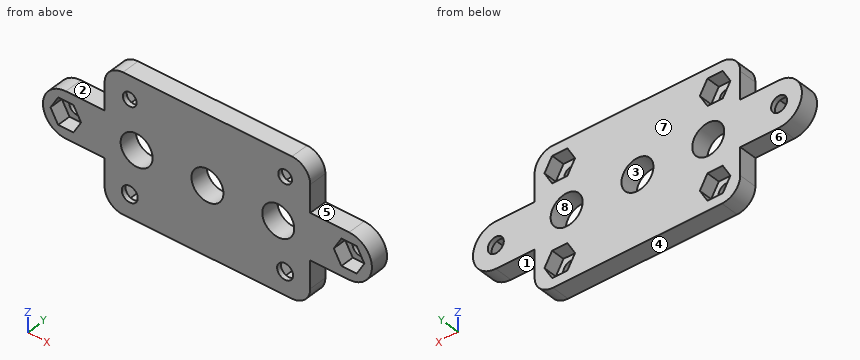
from build123d import *

# Parameters (mm, degrees)
ESBO_O2_R                = 1.75
ESBO_O2_R_2              = 1.5
ESBO_O2_R_3              = 3.5
RESSALTO_EXTRUS_O1_DEPTH = 4
CORTE_EXTRUS_O1_DEPTH    = 3
FILETE1_R                = 4
CORTE_EXTRUS_O2_DEPTH    = 3


with BuildPart() as part:
    # Esboço2 → Ressalto-extrusão1 (new body)
    with BuildSketch(Plane(origin=(0, 0, 0), x_dir=(1, 0, 0), z_dir=(0, 1, 0))):
        with BuildLine():
            Line((-22.5, -15), (22.5, -15))
            Line((22.5, -15), (22.5, -5))
            Line((22.5, -5), (31, -5))
            ThreePointArc((31, -5), (36, 0), (31, 5))
            Line((31, 5), (22.5, 5))
            Line((22.5, 5), (22.5, 15))
            Line((22.5, 15), (-22.5, 15))
            Line((-22.5, 15), (-22.5, 5))
            Line((-22.5, 5), (-31, 5))
            ThreePointArc((-31, 5), (-36, 0), (-31, -5))
            Line((-31, -5), (-22.5, -5))
            Line((-22.5, -5), (-22.5, -15))
        make_face()
        with Locations(Location((17, 10, 0), (0, 0, 270))):
            Circle(ESBO_O2_R, mode=Mode.SUBTRACT)
        with Locations(Location((17, -10, 0), (0, 0, 270))):
            Circle(ESBO_O2_R_2, mode=Mode.SUBTRACT)
        with Locations(Location((-17, -10, 0), (0, 0, 90))):
            Circle(ESBO_O2_R_2, mode=Mode.SUBTRACT)
        with Locations(Location((-17, 10, 0), (0, 0, 90))):
            Circle(ESBO_O2_R, mode=Mode.SUBTRACT)
        with Locations(Location((31, 0, 0), (0, 0, 270))):
            Circle(ESBO_O2_R, mode=Mode.SUBTRACT)
        with Locations(Location((-31, 0, 0), (0, 0, 90))):
            Circle(ESBO_O2_R, mode=Mode.SUBTRACT)
        with Locations(Location((0, 0, 0), (0, 0, 270))):
            Circle(ESBO_O2_R_3, mode=Mode.SUBTRACT)
        with Locations(Location((15.5, 0, 0), (0, 0, 270))):
            Circle(ESBO_O2_R_3, mode=Mode.SUBTRACT)
        with Locations(Location((-15.5, 0, 0), (0, 0, 90))):
            Circle(ESBO_O2_R_3, mode=Mode.SUBTRACT)
    extrude(amount=RESSALTO_EXTRUS_O1_DEPTH)

    # Esboço3 → Corte-extrusão1 (cut)
    with BuildSketch(Plane(origin=(0, 4, 0), x_dir=(1, 0, 0), z_dir=(0, 1, 0))):
        Polygon((-13.651368439, 10), (-15.325684219, 12.9), (-18.674315781, 12.9), (-20.348631561, 10), (-18.674315781, 7.1), (-15.325684219, 7.1), align=None)
        Polygon((-20.348631561, -10), (-18.674315781, -7.1), (-15.325684219, -7.1), (-13.651368439, -10), (-15.325684219, -12.9), (-18.674315781, -12.9), align=None)
        Polygon((18.674315781, -7.1), (15.325684219, -7.1), (13.651368439, -10), (15.325684219, -12.9), (18.674315781, -12.9), (20.348631561, -10), align=None)
        Polygon((15.325684219, 7.1), (13.651368439, 10), (15.325684219, 12.9), (18.674315781, 12.9), (20.348631561, 10), (18.674315781, 7.1), align=None)
    extrude(amount=-CORTE_EXTRUS_O1_DEPTH, mode=Mode.SUBTRACT)

    # Filete1
    filete1_edges = [part.edges().sort_by_distance(p)[0] for p in [
        (22.5, 2, 15),
        (-22.5, 2, 15),
        (-22.5, 2, -15),
        (22.5, 2, -15),
    ]]
    fillet(filete1_edges, radius=FILETE1_R)

    # Esboço6 → Corte-extrusão2 (cut)
    with BuildSketch(Plane.XZ):
        Polygon((-27.651368439, 0), (-29.325684219, 2.9), (-32.674315781, 2.9), (-34.348631561, 0), (-32.674315781, -2.9), (-29.325684219, -2.9), align=None)
        Polygon((29.325684219, -2.9), (27.651368439, 0), (29.325684219, 2.9), (32.674315781, 2.9), (34.348631561, 0), (32.674315781, -2.9), align=None)
    extrude(amount=-CORTE_EXTRUS_O2_DEPTH, mode=Mode.SUBTRACT)


solid = part.part
The model under review builds one solid part; all positions refer to its coordinate system, in mm. Face numbers are marked on the shaded views. A direction names the side the tool comes from. Give positions to 0.01 mm unless a question says otherwise; leave off trailing zeros. Write each loop counter-clockwise with the first axis right and the second up, starting at its lowest first coordinate (ties: lowest second). Pieces come first, ordered by that corner, then holes.
1. Wall thickness on L1, parallel to X at y = 0.35, z = 10; L2, parallel to X at y = 3.05, z = 0; L3, parallel to X at y = 1.05, z = 0: over which ranges is each line inside the solid? List them lowest first.
2. Draft analysis for pull direction Z (two halves, no side actions). For the marked faces 6, 7 and 8, state which applies: +Z half, -Z half, draft (parallel to the pull), parting line (faces both ways), or undercut.
3. Add section A-A, the plane x = -17. Write out the cut boundary in (y, z), plus the area to 3 significant figures.
4. Tool access review of the marked faces 1, 2, 3, 4 and 5: name each direction out of +Z, -Z, +X, -X, +Y, -Y from which nothing blocks a thin tool from reaching the whole face with its end or side.
5. Add section B-B, the plane x = -1.5. Write out the cut boundary in (y, z), plus the area to 3 significant figures.
6. For P1, Ø4.5, axis at x = -17, z = -10.5, coming from the +Y side; P2, Ø1.2, axis at y = 2, z = 9.5, coming from the -X side; P3, Ø2, axis at x = 27, y = 2.5, coming from the -Z side; P4, Ø3, axis at x = -17, z = -10, coming from the -Y side, all flat-tipped, find the tip position at first contact; note any pin that passes through.
7. Add section C-C, the plane x = -28.5. Write out the cut boundary in (y, z).
Worked answers:
1. L1: x = -22.5 to -18.5, -15.5 to 15.5, 18.5 to 22.5
1. L2: x = -36 to -32.75, -29.25 to -19, -12 to -3.5, 3.5 to 12, 19 to 29.25, 32.75 to 36
1. L3: x = -36 to -34.35, -27.65 to -19, -12 to -3.5, 3.5 to 12, 19 to 27.65, 34.35 to 36
2. face 6: -Z half
2. face 7: draft
2. face 8: undercut
3. outline: (0, -15) - (4, -15) - (4, -12.9) - (1, -12.9) - (1, -11.75) - (0, -11.75) - close; (0, -8.25) - (1, -8.25) - (1, -7.1) - (4, -7.1) - (4, -3.16) - (0, -3.16) - close; (0, 3.16) - (4, 3.16) - (4, 7.1) - (1, 7.1) - (1, 8.5) - (0, 8.5) - close; (0, 11.5) - (1, 11.5) - (1, 12.9) - (4, 12.9) - (4, 15) - (0, 15) - close
3. area: 53.4 mm2
4. face 1: -Z, +X, +Y, -Y
4. face 2: +Z, -X, +Y, -Y
4. face 3: +Y, -Y
4. face 4: -Z, +X, -X, +Y, -Y
4. face 5: +Z, +X, +Y, -Y
5. outline: (0, -15) - (4, -15) - (4, -3.16) - (0, -3.16) - close; (0, 3.16) - (4, 3.16) - (4, 15) - (0, 15) - close
5. area: 94.7 mm2
6. P1: stops at y = 1
6. P2: stops at x = -22.5
6. P3: stops at z = -5
6. P4: passes through
7. outline: (0, -5) - (4, -5) - (4, 5) - (0, 5) - (0, 1.47) - (3, 1.47) - (3, -1.47) - (0, -1.47) - close
